from build123d import *

# Parameters (mm, degrees)
F1_DEPTH = 120
F2_R     = 5
F3_R     = 1.99999


# Not quite as in the source:
# - a fillet or chamfer is up to 0.001 mm smaller than in the source, because OpenCascade refuses the exact size


with BuildPart() as f1:
    # F0 (on Front) → F1 (new body)
    with BuildSketch(Plane.XZ):
        Polygon((1, 60), (0, 60), (-1, 60), (-1, 2), (-31, 2), (-31, 0), (0, 0), (31, 0), (31, 2), (1, 2), align=None)
    extrude(amount=F1_DEPTH)

    # F2
    f2_edges = [f1.edges().sort_by_distance(p)[0] for p in [
        (-1, -60, 2),
        (1, -60, 2),
    ]]
    fillet(f2_edges, radius=F2_R)

    # F3 (radius 2 in the source; OpenCascade refuses exactly that, so slightly less here)
    f3_edges = [f1.edges().sort_by_distance(p)[0] for p in [
        (31, -60, 2),
        (-31, -60, 2),
    ]]
    fillet(f3_edges, radius=F3_R)


solid = f1.part
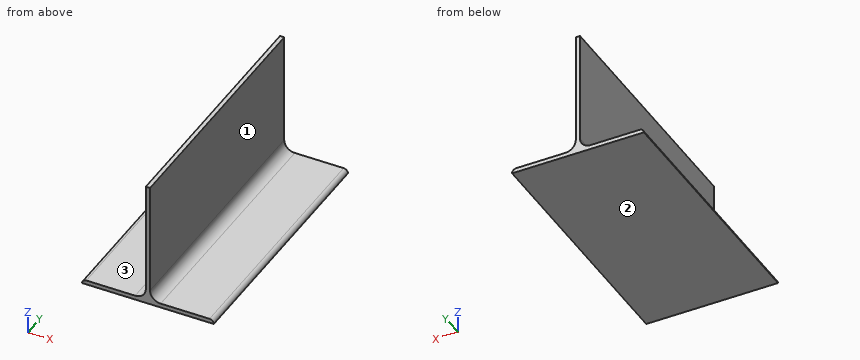
Input: part model. Units: mm. Frame: model coordinates. Face numbers are marked on the shaded views. A direction names the side the tool comes from. Give positions to 0.01 mm unless a question says otherwise; leave off trailing zeros. Order: outer loops, then holes, each group sorted by start corner. A loop starts at its lowest first (then second) coordinate and runs counter-clockwise, first axis right, second up. Notation, with made-up numbers: M 36,63 L 85,63 A22 cw 85,96 Z; hole C 45,65 d5. An arc over 180 degrees is marked long. Answer as a JSON object with one key per item and string values.
1. Cut plane C-C, the plane z = 39. Output: boundary loops of the cut face in (x, y), and give its area (3 significant figures).
Result sheet:
{"outline": "M -1,-120 L 1,-120 L 1,0 L -1,0 Z", "area": "240 mm²"}
2. Cut plane B-B, the plane x = 21. Output: boundary loops of the cut face in (y, z).
Result sheet:
{"outline": "M -120,0 L 0,0 L 0,2 L -120,2 Z"}
3. Reachability of the marked faces 1, 2 and 3 from +Z, -Z, +X, -X, +Y, -Y: full face, straight path, thin tool, end or side. Return the list, or none.
Result sheet:
{"face 1": "+Z, +X, +Y, -Y", "face 2": "-Z, +X, -X, +Y, -Y", "face 3": "+Z, -X, +Y, -Y"}
4. First-contact query: P1, Ø11.5, axis at x = -13.5, y = -69.5, coming from the +Z side; P2, Ø10, axis at y = -88.5, z = 30, coming from the +X side; P3, Ø1, axis at y = -56.5, z = 54, coming from the -X side. Flat tips, straight axial feed; report the tip coordinate or a pass-through.
Result sheet:
{"P1": "z = 2", "P2": "x = 1", "P3": "x = -1"}
5. Ray query, line 1 (Z direction, x = 20, y = -42.5); line 2 (X direction, y = -110.5, z = 9.5); line 3 (X direction, y = -71, z = 5.5). Return the intervals inside material, ascending. Write a range as [from, to].
Result sheet:
{"line 1": "[0, 2]", "line 2": "[-1, 1]", "line 3": "[-1.23, 1.23]"}
